Verification items for the finished model (mm, model axes). Round coordinates to 2 decimals unless told otherwise and drop trailing zeros. Write each loop counter-clockwise with the first axis right and the second up, starting at its lowest first coordinate (ties: lowest second). Pieces come first, ordered by that corner, then holes. Notation, with made-up numbers: M 72.25,-0.5 L 106.25,-0.5 A9 ccw 106.25,8.5 Z; hole C 21,46.25 d10. An arc over 180 degrees is marked long. One line per item, written item: value. Start each with the question number.
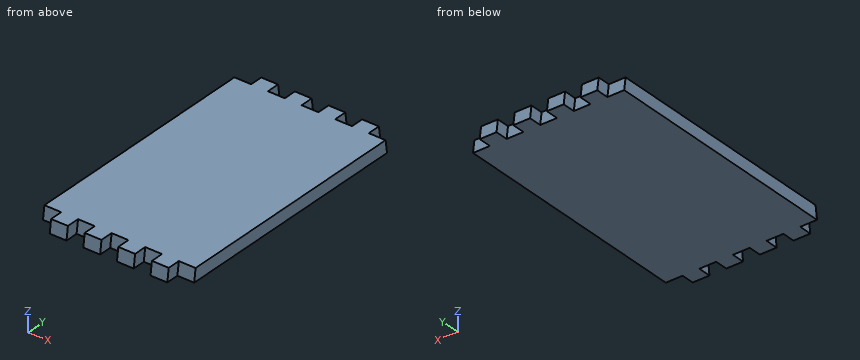
from build123d import *

# Parameters (mm, degrees)
F0_W     = 214.3125
F0_H     = 384.175
F1_DEPTH = 18.034
F3_DEPTH = 214.3125
F6_DEPTH = 18.034


# Not quite as in the source:
# - a pattern or mirror of a feature is missing from the dataset's text; its kind, count and spacing are read off the source's solid


with BuildPart() as f1:
    # F0 (on Top) → F1 (new body)
    with BuildSketch(Plane.XY):
        Rectangle(F0_W, F0_H)
    extrude(amount=F1_DEPTH)

    # F2 (on face) → F3 (cut, through all)
    with BuildSketch(Plane(origin=(-107.15625, 0, 0), x_dir=(0, -1, 0), z_dir=(-1, 0, 0))):
        Polygon((-204.7875, 0), (-192.0875, 0), (-189.552986587, 18.034), (-204.7875, 18.034), align=None)
    f3 = extrude(amount=-F3_DEPTH, mode=Mode.SUBTRACT)

    # F3_copies: F3 across plane
    add(f3.mirror(Plane(origin=(0, 0, 0), x_dir=(0, 0, -1), z_dir=(0, -1, 0))), mode=Mode.SUBTRACT)

    # F5 (on offset) → F6 (cut)
    with BuildSketch(Plane(origin=(0, 188.3669280093, 26.4732452927), x_dir=(-1, 0, 0), z_dir=(0, 0.9902680687, 0.139173101))):
        Polygon((-83.34375, -1.3334130307), (-107.15625, -1.3334130307), (-107.15625, -26.7334130307), (-107.15625, -33.0834130307), (107.15625, -33.0834130307), (107.15625, -26.7334130307), (107.15625, -1.3334130307), (83.34375, -1.3334130307), (83.34375, -26.7334130307), (59.53125, -26.7334130307), (59.53125, -1.3334130307), (35.71875, -1.3334130307), (35.71875, -26.7334130307), (11.90625, -26.7334130307), (11.90625, -1.3334130307), (-11.90625, -1.3334130307), (-11.90625, -26.7334130307), (-35.71875, -26.7334130307), (-35.71875, -1.3334130307), (-59.53125, -1.3334130307), (-59.53125, -26.7334130307), (-83.34375, -26.7334130307), align=None)
    f6 = extrude(amount=-F6_DEPTH, mode=Mode.SUBTRACT)

    # F6_copies: F6 across plane
    add(f6.mirror(Plane(origin=(0, 0, 0), x_dir=(0, 0, -1), z_dir=(0, -1, 0))), mode=Mode.SUBTRACT)


solid = f1.part
1) Thickness scan on line 1 (Y direction, x = 20.5, z = 15); line 2 (Y direction, x = -29.5, z = 11). Record the ranges inside material, lowest first.
2) Cross-section at A-A (x = 54). Record the boundary of the cut face in (y, z).
3) Gauge pin test, flat ends, axial feed: pin 1 Ø5.5 at (y, z) = (-178, 7.5) entering from -X; pin 2 Ø5.5 at (y, z) = (-183.5, 9) entering from +X; pin 3 Ø1 at (x, z) = (-40, 15) entering from -Y. Record the tip position at first contact, or that the pin passes through.
Results below:
1. line 1: y = -189.98 to 189.98
1. line 2: y = -190.54 to 190.54
2. outline: M -173.88,0 L 173.88,0 L 171.34,18.03 L -171.34,18.03 Z
3. pin 1: stops at x = -83.34
3. pin 2: stops at x = 83.34
3. pin 3: stops at y = -171.84
